from build123d import *

# Parameters (mm, degrees)
F0_R          = 48.683007
F0_R_2        = 34.725428
F1_DEPTH      = 50.8
F3_DEPTH      = 19.05
F5_DEPTH      = 12.7
F5_DEPTH_BACK = 12.7


with BuildPart() as f1:
    # F0 (on Top) → F1 (new body)
    with BuildSketch(Plane.XY):
        Circle(F0_R)
        Circle(F0_R_2, mode=Mode.SUBTRACT)
    extrude(amount=F1_DEPTH)

    # F2 (on Top) → F3 (join)
    with BuildSketch(Plane.XY):
        with BuildLine():
            ThreePointArc((-12.464464, -39.019189), (-40.947813, -1.066114), (-14.478001, 38.317718))
            Line((-14.478001, 38.317718), (-106.571145, 38.317718))
            Line((-106.571145, 38.317718), (-106.571145, -39.019189))
            Line((-106.571145, -39.019189), (-12.464464, -39.019189))
        make_face()
    extrude(amount=F3_DEPTH)

    # F4 (on Front) → F5 (join, two sides)
    with BuildSketch(Plane.XZ) as f5_sk:
        Polygon((-46.427574, 16.981715), (-46.427574, 48.332572), (-95.195569, 16.981715), align=None)
    extrude(amount=F5_DEPTH)
    extrude(f5_sk.sketch, amount=-F5_DEPTH_BACK)


solid = f1.part
Geometry: final body of the model. Coordinates: model frame, mm. A direction names the side the tool comes from. Round coordinates to 2 decimals unless told otherwise and drop trailing zeros. Order: outer loops, then holes, each group sorted by start corner. A loop starts at its lowest first (then second) coordinate and runs counter-clockwise, first axis right, second up.
Q1. Material intervals for probe 1 along Y at (x, z) = (0, 39); probe 2 along Y at (x, z) = (-17, 44.5); probe 3 along X at (y, z) = (24.5, 46.5), sorted ascending.
Result sheet:
probe 1: y = -48.68 to -34.73, 34.73 to 48.68
probe 2: y = -45.62 to -30.28, 30.28 to 45.62
probe 3: x = -42.07 to -24.61, 24.61 to 42.07
Q2. Section C-C, the plane z = 16.5. Output: boundary loops of the cut face in (x, y), and give its area (3 significant figures).
Result sheet:
outline: (-106.57, -39.02) - (-29.11, -39.02) arc R48.68 ccw (long way) to (-30.03, 38.32) - (-106.57, 38.32) - close; hole circle Ø69.45 at (0, 0)
area: 8,580 mm2
Q3. Section D-D, the plane x = -81. Output: boundary loops of the cut face in (y, z).
Result sheet:
outline: (-39.02, 0) - (38.32, 0) - (38.32, 19.05) - (12.7, 19.05) - (12.7, 26.11) - (-12.7, 26.11) - (-12.7, 19.05) - (-39.02, 19.05) - close
Q4. Access query for faces 1 (the face through (-60, 12.7, 27)), 2 (the face through (-12, 33, 50.8)), 3 (the face through (-68, 38.318, 9)), 4 (the face through (-60, -12.7, 27)), 5 (the face through (-77, 17, 19.05)). Directions: +Z, -Z, +X, -X, +Y, -Y. A direction counts if a zero-diameter tool reaches every point of the face in a straight line with its end or side. Return the directions, or none.
Result sheet:
face 1: +Z, -X, +Y
face 2: +Z, +X, -X, +Y, -Y
face 3: +Z, -Z, -X, +Y
face 4: +Z, -X, -Y
face 5: +Z, -X
Q5. Section A-A, the plane x = 0. Output: boundary loops of the cut face in (y, z), and give its area (3 significant figures).
Result sheet:
outline: (-48.68, 0) - (-34.73, 0) - (-34.73, 50.8) - (-48.68, 50.8) - close; (34.73, 0) - (48.68, 0) - (48.68, 50.8) - (34.73, 50.8) - close
area: 1,420 mm2
Q6. Section B-B, the plane y = -20. Output: boundary loops of the cut face in (x, z), and give its area (3 significant figures).
Result sheet:
outline: (-106.57, 0) - (-28.39, 0) - (-28.39, 50.8) - (-44.39, 50.8) - (-44.39, 19.05) - (-106.57, 19.05) - close; (28.39, 0) - (44.39, 0) - (44.39, 50.8) - (28.39, 50.8) - close
area: 2,810 mm2
Q7. Mould query, pull axis Y, two halves, no side actions, for faces 6 (the face through (46.435, 14.623, 25.044)), 7 (the face through (33.12, 10.43, 25.04)), 8 (the face through (-68, -39.019, 9)), 9 (the face through (-106.571, 0, 9)). Classes: released by +Y, released by -Y, zero draft, split by the parting line, or undercut.
Result sheet:
face 6: split by the parting line
face 7: undercut
face 8: released by -Y
face 9: zero draft
Q8. Pin query (flat end, axial travel): pin 1 (14.5 mm diameter, centred on x = -77, z = 32, fed in from -Y); pin 2 (8.5 mm diameter, centred on x = -59, z = 39.5, fed in from +Y); pin 3 (10 mm diameter, centred on x = -60.5, z = 22, fed in from -Y). Return the tip coordinate at first contact, or that it passes through.
Result sheet:
pin 1: stops at y = -12.7
pin 2: stops at y = 12.7
pin 3: stops at y = -39.02
